Source: three-view drawing plus pictorial views. Frame: mm from the lowest corner of the part. A direction names the side the tool comes from. Give positions to 0.01 mm unless a question says otherwise; leave off trailing zeros. Write each loop counter-clockwise with the first axis right and the second up, starting at its lowest first coordinate (ties: lowest second). Pieces come first, ordered by that corner, then holes. Notation, with made-up numbers: (33.5, 38) -> (74.5, 38) arc R28 cw to (74.5, 70) -> close; hole circle Ø5 at (21.25, 50.25). An arc over 180 degrees is marked (long way). Answer in a Markdown table with one row per item. Add a question column.
Item 1: Material intervals for probe 1 along Y at (x, z) = (50.5, 13) (1 decimal); probe 2 along Z at (x, y) = (54, 17); probe 3 along X at (y, z) = (10.75, 17.25) (1 decimal), sorted ascending. Write a range as from..to.
Item 2: First-contact query: P1, Ø1, axis at y = 4, z = 11, coming from the -X side; P2, Ø1.1, axis at x = 32.5, y = 2, coming from the +Z side; P3, Ø10, axis at x = 31.5, y = 3.5, coming from the +Z side; P4, Ø3, axis at x = 48.5, z = 12.5, coming from the +Y side. Flat tips, straight axial feed; report the tip coordinate or a pass-through.
Item 3: Section query B-B on z = 11.75. Output: boundary loops of the cut face in (x, y) (1 decimal), plus the area to 3 significant figures.
Item 4: Section query C-C on y = 5.5. Output: boundary loops of the cut face in (x, z).
Item 5: Access query for the marked faces 1, 2 and 3. Directions: +Z, -Z, +X, -X, +Y, -Y. A direction counts if a zero-diameter tool reaches every point of the face in a straight line with its end or side. Return the directions, or none.
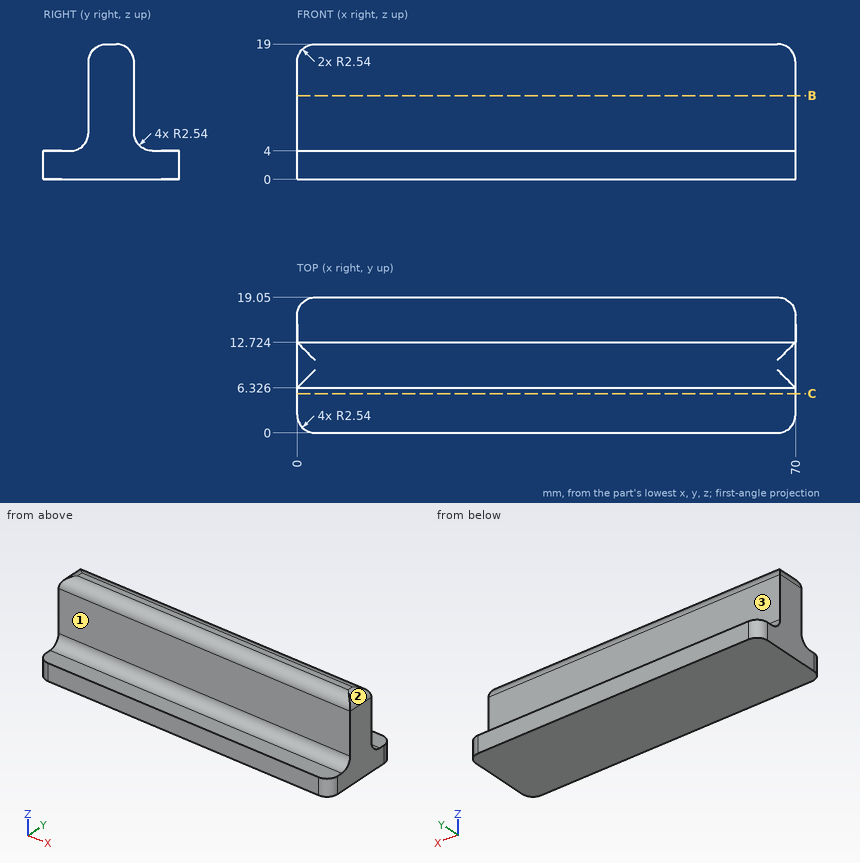
Findings below:
| question | item | result |
|---|---|---|
| 1 | probe 1 | y = 6.3..12.7 |
| 1 | probe 2 | z = 0..4 |
| 1 | probe 3 | x = 0.1..69.9 |
| 2 | P1 | passes through |
| 2 | P2 | stops at z = 4 |
| 2 | P3 | stops at z = 18.97 |
| 2 | P4 | stops at y = 12.72 |
| 3 | outline | (0, 6.3) -> (70, 6.3) -> (70, 12.7) -> (0, 12.7) -> close |
| 3 | area | 448 mm^2 |
| 4 | outline | (0, 0) -> (70, 0) -> (70, 4.67) -> (0, 4.67) -> close |
| 5 | face 1 | +Z, +X, -X, -Y |
| 5 | face 2 | +Z, +X, +Y, -Y |
| 5 | face 3 | +Z, +X, -X, +Y |
